Input: part model. Units: mm. Frame: model coordinates. A direction names the side the tool comes from. Coordinates: 2 decimals unless noted, no trailing zeros. Loops run counter-clockwise (first coordinate to the right, second up) from the corner with the lowest first, then second, coordinate; pieces in that order, holes last. Notation, with made-up numbers: M 83.25,-26 L 112.25,-26 A16 ccw 112.25,-16 Z; hole C 45,58.25 d2. An arc over 180 degrees is marked long. Use a Markdown table: item, result. Add a question column.
1. Section A-A on z = 193.5. Output: boundary loops of the cut face in (x, y).
2. Line query: L1, parallel to X at y = 1.45, z = 130; L2, parallel to Y at x = -5, z = 196; L3, parallel to X at y = 2.4, z = 130. Output: solid intervals per line, ascending. Write a range as [from, to].
3. Pin query (flat end, axial travel): pin 1 (1.8 mm diameter, centred on x = 0.5, z = 131, fed in from +Y). Return the tip coordinate at first contact, or that it passes through.
4. Section B-B on y = -2.25. State how many separate pieces and enclosed holes the cut face has, then the cut area to 3 significant figures.
5. Set-up query: faces 1 (the cylindrical face through (0.9, 1.78, 157.86)), 2 (the cylindrical face through (-0.67, -2.23, 106.62)). Return all of +Z, -Z, +X, -X, +Y, -Y with unobstructed straight access to the full face (end or side cutting, diameter ignored); none if empty.
6. Section C-C on z = 155. Output: boundary loops of the cut face in (x, y).
7. Draft query along Z for faces 3 (the flat face through (-4, 4, 106)), 4 (the flat face through (0, 0, 215)), 5 (the flat face through (0, 0, 0)), 6 (the cylindrical face through (0.077, -2.226, 78.253)). Return one class per face: +Z half, -Z half, draft (parallel to the pull), parting line (faces both ways), or undercut.
```python
from build123d import *

# Parameters (mm, degrees)
BOSS_EXTRUDE1_DEPTH = 215
SKETCH2_R           = 3
CUT_EXTRUDE1_DEPTH  = 4.5
SKETCH3_R           = 1.75
CUT_EXTRUDE2_DEPTH  = 216.2324325


with BuildPart() as part:
    # Sketch1 → Boss-Extrude1 (new body)
    with BuildSketch(Plane.XY):
        with BuildLine():
            Line((-5.6, 4), (5.6, 4))
            ThreePointArc((5.6, 4), (5.882842712, 3.882842712), (6, 3.6))
            Line((6, 3.6), (6, 2.8))
            Line((6, 2.8), (5.2, 2))
            Line((5.2, 2), (4.4, 2))
            Line((4.4, 2), (4.4, 1))
            Line((4.4, 1), (5.2, 1))
            Line((5.2, 1), (6, 0.2))
            Line((6, 0.2), (6, -3.6))
            ThreePointArc((6, -3.6), (5.882842712, -3.882842712), (5.6, -4))
            Line((5.6, -4), (-5.6, -4))
            ThreePointArc((-5.6, -4), (-5.882842712, -3.882842712), (-6, -3.6))
            Line((-6, -3.6), (-6, 0.2))
            Line((-6, 0.2), (-5.2, 1))
            Line((-5.2, 1), (-4.4, 1))
            Line((-4.4, 1), (-4.4, 2))
            Line((-4.4, 2), (-5.2, 2))
            Line((-5.2, 2), (-6, 2.8))
            Line((-6, 2.8), (-6, 3.6))
            ThreePointArc((-6, 3.6), (-5.882842712, 3.882842712), (-5.6, 4))
        make_face()
    extrude(amount=BOSS_EXTRUDE1_DEPTH)

    # Sketch2 → Cut-Extrude1 (cut)
    with BuildSketch(Plane(origin=(0, 4, 0), x_dir=(1, 0, 0), z_dir=(0, 1, 0))):
        with Locations(Location((0, -205, 0), (0, 0, 270))):
            Circle(SKETCH2_R)
        with Locations(Location((0, -180, 0), (0, 0, 270))):
            Circle(SKETCH2_R)
        with Locations(Location((0, -155, 0), (0, 0, 270))):
            Circle(SKETCH2_R)
        with Locations(Location((0, -130, 0), (0, 0, 270))):
            Circle(SKETCH2_R)
        with Locations(Location((0, -105, 0), (0, 0, 270))):
            Circle(SKETCH2_R)
        with Locations(Location((0, -80, 0), (0, 0, 270))):
            Circle(SKETCH2_R)
        with Locations(Location((0, -55, 0), (0, 0, 270))):
            Circle(SKETCH2_R)
        with Locations(Location((0, -30, 0), (0, 0, 270))):
            Circle(SKETCH2_R)
        with Locations(Location((0, -5, 0), (0, 0, 270))):
            Circle(SKETCH2_R)
        with Locations((0, 20)):
            Circle(SKETCH2_R)
        with Locations((0, 45)):
            Circle(SKETCH2_R)
        with Locations((0, 70)):
            Circle(SKETCH2_R)
        with Locations((0, 95)):
            Circle(SKETCH2_R)
        with Locations((0, 120)):
            Circle(SKETCH2_R)
        with Locations((0, 145)):
            Circle(SKETCH2_R)
        with Locations((0, 170)):
            Circle(SKETCH2_R)
        with Locations((0, 195)):
            Circle(SKETCH2_R)
        with Locations((0, 220)):
            Circle(SKETCH2_R)
    extrude(amount=-CUT_EXTRUDE1_DEPTH, mode=Mode.SUBTRACT)

    # Sketch3 → Cut-Extrude2 (cut, through all)
    with BuildSketch(Plane(origin=(0, 4, 0), x_dir=(1, 0, 0), z_dir=(0, 1, 0))):
        with Locations(Location((0, -205.001504258, 0), (0, 0, 270))):
            Circle(SKETCH3_R)
        with Locations(Location((0, -180.001504258, 0), (0, 0, 270))):
            Circle(SKETCH3_R)
        with Locations(Location((0, -155.001504258, 0), (0, 0, 270))):
            Circle(SKETCH3_R)
        with Locations(Location((0, -130.001504258, 0), (0, 0, 270))):
            Circle(SKETCH3_R)
        with Locations(Location((0, -105.001504258, 0), (0, 0, 270))):
            Circle(SKETCH3_R)
        with Locations(Location((0, -80.001504258, 0), (0, 0, 270))):
            Circle(SKETCH3_R)
        with Locations(Location((0, -55.001504258, 0), (0, 0, 270))):
            Circle(SKETCH3_R)
        with Locations(Location((0, -30.001504258, 0), (0, 0, 270))):
            Circle(SKETCH3_R)
        with Locations(Location((0, -5.001504258, 0), (0, 0, 270))):
            Circle(SKETCH3_R)
        with Locations((0, 19.998495742)):
            Circle(SKETCH3_R)
        with Locations((0, 44.998495742)):
            Circle(SKETCH3_R)
        with Locations((0, 69.998495742)):
            Circle(SKETCH3_R)
        with Locations((0, 94.998495742)):
            Circle(SKETCH3_R)
        with Locations((0, 119.998495742)):
            Circle(SKETCH3_R)
        with Locations((0, 144.998495742)):
            Circle(SKETCH3_R)
    extrude(amount=-CUT_EXTRUDE2_DEPTH, mode=Mode.SUBTRACT)


solid = part.part
```
Answers below:
| question | item | result |
|---|---|---|
| 1 | outline | M -6,-3.6 A0.4 ccw -5.6,-4 L 5.6,-4 A0.4 ccw 6,-3.6 L 6,0.2 L 5.2,1 L 4.4,1 L 4.4,2 L 5.2,2 L 6,2.8 L 6,3.6 A0.4 ccw 5.6,4 L -5.6,4 A0.4 ccw -6,3.6 L -6,2.8 L -5.2,2 L -4.4,2 L -4.4,1 L -5.2,1 L -6,0.2 Z |
| 2 | L1 | x = [-4.4, -3], [3, 4.4] |
| 2 | L2 | y = [-4, 1], [2, 4] |
| 2 | L3 | x = [-5.6, -3], [3, 5.6] |
| 3 | pin 1 | stops at y = -0.5 |
| 4 | separate pieces | 1 |
| 4 | enclosed holes | 9 |
| 4 | area | 2,490 mm² |
| 5 | face 1 | +Y |
| 5 | face 2 | +Y, -Y |
| 6 | outline | M -6,-3.6 A0.4 ccw -5.6,-4 L -1.75,-4 L -1.75,-0.5 L -3,-0.5 L -3,4 L -5.6,4 A0.4 ccw -6,3.6 L -6,2.8 L -5.2,2 L -4.4,2 L -4.4,1 L -5.2,1 L -6,0.2 Z; M 1.75,-4 L 5.6,-4 A0.4 ccw 6,-3.6 L 6,0.2 L 5.2,1 L 4.4,1 L 4.4,2 L 5.2,2 L 6,2.8 L 6,3.6 A0.4 ccw 5.6,4 L 3,4 L 3,-0.5 L 1.75,-0.5 Z |
| 7 | face 3 | draft |
| 7 | face 4 | +Z half |
| 7 | face 5 | -Z half |
| 7 | face 6 | undercut |
